Build history of the part. All positions in model axes, mm. A direction names the side the tool comes from. Give positions to 0.01 mm unless a question says otherwise; leave off trailing zeros. Order: outer loops, then holes, each group sorted by start corner. A loop starts at its lowest first (then second) coordinate and runs counter-clockwise, first axis right, second up. Notation, with made-up numbers: M 85.5,86 L 138.5,86 A15 cw 138.5,94 Z; hole C 64.25,27.25 d5. An arc over 180 degrees is marked long. Use CSV: the item, a comma, the result in double quotes. Start each with the question number.
Item 1: Which spindle directions (+Z, -Z, +X, -X, +Y, -Y) get a long thin tool onto all of the face, cutting with end or side? Do faces 1 (the flat face through (21, 1, 0)), 2 (the cylindrical face through (0.69, -93.66, 3.22)), 3 (the cylindrical face through (84.795, 26.703, 4.785)). Say none if no direction does.
Item 2: Two-plate mould, pull along X, no slides. Class faces 4 (the flat face through (-1, -19, 3.175)), 5 (the flat face through (67, -60, 6.35)), 6 (the cylindrical face through (-22.025, -99.184, 3.131)): pulls with the +X half, pulls with the -X half, needs draft (parallel to the pull), parting line crosses it, or undercut.
Item 3: Wall check: line 1 along Y through (x, z) = (0, 4.35); line 2 along Y through (x, z) = (0, 1.3); line 3 along Z through (x, y) = (37, 77) (3 decimals). Give the ranges that are in metal, low to high.
Item 4: Pin check, flat tips, straight feed: P1, Ø1, axis at x = -17, y = -37, coming from the +Z side (3 decimals); P2, Ø11.5, axis at x = 0, y = 0, coming from the +Z side (3 decimals); P3, Ø1.5, axis at y = -30.5, z = 5.5, coming from the +X side. Stop position of each tip, or through.
Item 5: Band-saw the part on B-B on x = 0. Give the number of separate pieces and of enclosed holes in the cut face, plus the area to 3 significant figures.
Item 6: Band-saw the part on A-A on y = 0. Write the cut outline in (x, z) (3 decimals), plus the area to 3 significant figures.
Item 7: Band-saw the part on C-C on z = 4.5. Write the cut outline in (x, y) (1 decimal), plus the area to 3 significant figures.
Item 8: Band-saw the part on D-D on y = 43.5. Write the cut outline in (x, z) (3 decimals), plus the area to 3 significant figures.
from build123d import *

# Parameters (mm, degrees)
SKETCH1_R      = 101.6
RADIUS_DEPTH   = 6.35
SKETCH4_R      = 88.9
EXTRUDE4_DEPTH = 3.175
EXTRUDE5_DEPTH = 144.824345992
SKETCH14_R     = 6.35
EXTRUDE6_DEPTH = 6.35


with BuildPart() as part:
    # Sketch1 → Radius (new body)
    with BuildSketch(Plane.XY):
        Circle(SKETCH1_R)
    extrude(amount=RADIUS_DEPTH)

    # Sketch4 → Extrude4 (cut)
    with BuildSketch(Plane.XY.offset(6.35)):
        Circle(SKETCH4_R)
    extrude(amount=-EXTRUDE4_DEPTH, mode=Mode.SUBTRACT)

    # Sketch7 → Extrude5 (cut, through all)
    with BuildSketch(Plane.XY.offset(6.35)):
        with BuildLine():
            ThreePointArc((46.83125, -81.114104382), (0, -93.6625), (-46.83125, -81.114104382))
            ThreePointArc((-46.83125, -81.114104382), (-48.999815329, -81.69516971), (-48.41875, -83.863735039))
            ThreePointArc((-48.41875, -83.863735039), (0, -96.8375), (48.41875, -83.863735039))
            ThreePointArc((48.41875, -83.863735039), (48.999815329, -81.69516971), (46.83125, -81.114104382))
        make_face()
    extrude(amount=-EXTRUDE5_DEPTH, mode=Mode.SUBTRACT)

    # Sketch14 → Extrude6 (cut)
    with BuildSketch(Plane.XY.offset(3.175)):
        Circle(SKETCH14_R)
    extrude(amount=-EXTRUDE6_DEPTH, mode=Mode.SUBTRACT)


solid = part.part
Model answer:
1,face 1,"-Z, +X, -X, +Y, -Y"
1,face 2,"+Z, -Z"
1,face 3,"+Z"
2,face 4,"undercut"
2,face 5,"needs draft"
2,face 6,"parting line crosses it"
3,line 1,"y = -101.6 to -96.84, -93.66 to -88.9, 88.9 to 101.6"
3,line 2,"y = -101.6 to -96.84, -93.66 to -6.35, 6.35 to 101.6"
3,line 3,"z = 0 to 3.175"
4,P1,"stops at z = 3.175"
4,P2,"passes through"
4,P3,"stops at x = 97.15"
5,separate pieces,"3"
5,enclosed holes,"0"
5,area,"665 mm^2"
6,outline,"M -101.6,0 L -6.35,0 L -6.35,3.175 L -88.9,3.175 L -88.9,6.35 L -101.6,6.35 Z; M 6.35,0 L 101.6,0 L 101.6,6.35 L 88.9,6.35 L 88.9,3.175 L 6.35,3.175 Z"
6,area,"685 mm^2"
7,outline,"C 0,0 d203.2; hole C 0,0 d177.8; hole M -48.4,-83.9 A96.8 ccw 48.4,-83.9 A1.6 ccw 46.8,-81.1 A93.7 cw -46.8,-81.1 A1.6 ccw Z"
7,area,"7,280 mm^2"
8,outline,"M -91.817,0 L 91.817,0 L 91.817,6.35 L 77.53,6.35 L 77.53,3.175 L -77.53,3.175 L -77.53,6.35 L -91.817,6.35 Z"
8,area,"674 mm^2"
